Read the model definition and answer for the solid it produces. Units are mm, in the model's axes. A direction names the side the tool comes from. Round coordinates to 2 decimals unless told otherwise and drop trailing zeros. Order: outer loops, then holes, each group sorted by start corner. A loop starts at its lowest first (then second) coordinate and runs counter-clockwise, first axis right, second up. Notation, with made-up numbers: (2.5, 1) - (34.5, 1) arc R20 ccw to (34.5, 27) - close; hole circle Ø2 at (88, -31.75). An arc over 180 degrees is marked (long way). Answer as a JSON object with one key per item and string values. Group by question number.
Q1. A tool of negligible diameter and unlimited length cuts with its end or side. For faces 1 (the flat face through (-27, -12, 12)), 2 (the flat face through (-0.1, 10.2, 20)), 3 (the flat face through (27, -12, 12)), from which of +Z, -Z, +X, -X, +Y, -Y can it reach the whole face along a straight path? Write none if from no direction.
Q2. A cutting plane is placed at C-C on z = 1.5. Determine the outline of the cut face in (x, y).
Q3. A cutting plane is placed at D-D on y = -11. Determine the outline of the cut face in (x, z), and give its area (3 significant figures).
Q4. A cutting plane is placed at A-A on y = 0. Determine the outline of the cut face in (x, z), and give its area (3 significant figures).
Q5. A cutting plane is placed at B-B on x = 0. Determine the outline of the cut face in (y, z).
Q6. The mould has two halves that part along X. Classify faces 4 (the flat face through (30, -15, 12)), 5 (the flat face through (0, -8, 0)), 6 (the cylindrical face through (11.923, 3.755, 22.535)): pulls with the +X half, pulls with the -X half, needs draft (parallel to the pull), parting line crosses it, or undercut.
Q7. Given pin 1 Ø4 at (x, y) = (-21, -9.5) entering from +Z; pin 2 Ø1.5 at (x, z) = (10, 18.5) entering from +Y; pin 3 Ø7.5 at (x, y) = (-0.5, 3) entering from +Z; pin 4 Ø4 at (x, z) = (27.5, 9) entering from +Y, each flat-ended and moving along its own axis, determine where each tip first touches the part or whether it passes through.
Q8. Consider line 1 (Y direction, x = 0, z = 21.05); line 2 (Y direction, x = 0, z = 14.25); line 3 (Y direction, x = -26, z = 15.5). Determine where each line is inside the solid, lowest interval first.
```python
from build123d import *

# Parameters (mm, degrees)
F1_DEPTH       = 25
F2_R           = 10
F4_D           = 20
F4_DEPTH       = 22
F4_CBORE_D     = 25
F4_CBORE_DEPTH = 5
F4_TIP         = 6.0086061903


with BuildPart() as f1:
    # F0 (on Top) → F1 (new body)
    with BuildSketch(Plane.XY):
        with BuildLine():
            Line((9, -12), (-9, -12))
            ThreePointArc((-9, -12), (0, -15), (9, -12))
        make_face()
        with BuildLine():
            ThreePointArc((9, -12), (0, -15), (-9, -12))
            Line((-9, -12), (-30, -12))
            Line((-30, -12), (-30, -17))
            Line((-30, -17), (30, -17))
            Line((30, -17), (30, -12))
            Line((30, -12), (9, -12))
        make_face()
        with BuildLine():
            ThreePointArc((9, -12), (13.416407865, -6.7082039325), (15, 0))
            ThreePointArc((15, 0), (-6.7082039325, 13.416407865), (-9, -12))
            Line((-9, -12), (9, -12))
        make_face()
    extrude(amount=F1_DEPTH)

    # F2
    f2_edges = [f1.edges().sort_by_distance(p)[0] for p in [
        (-9, -12, 12.5),
        (9, -12, 12.5),
    ]]
    fillet(f2_edges, radius=F2_R)

    # F4
    with Locations(Plane.XY.offset(25)):
        with Locations((0, 0)):
            CounterBoreHole(F4_D / 2, F4_CBORE_D / 2, F4_CBORE_DEPTH, depth=F4_DEPTH)
            with Locations((0, 0, -(F4_DEPTH + F4_TIP / 2))):  # 118° drill point
                Cone(0, F4_D / 2, F4_TIP, mode=Mode.SUBTRACT)


solid = f1.part
```
Result set:
{
 "1": {"face 1": "+Z, -Z, -X, +Y", "face 2": "+Z", "face 3": "+Z, -Z, +X, +Y"},
 "2": {"outline": "(-30, -17) - (30, -17) - (30, -12) - (24.92, -12) arc R10 cw to (14.95, -1.2) arc R15 ccw (long way) to (-14.95, -1.2) arc R10 cw to (-24.92, -12) - (-30, -12) - close; hole circle Ø15.01 at (0, 0)"},
 "3": {"outline": "(-20.56, 0) - (20.56, 0) - (20.56, 25) - (5.94, 25) - (5.94, 20) - (-5.94, 20) - (-5.94, 25) - (-20.56, 25) - close", "area": "969 mm²"},
 "4": {"outline": "(-15, 0) - (-5.01, 0) - (-10, 3) - (-10, 20) - (-12.5, 20) - (-12.5, 25) - (-15, 25) - close; (5.01, 0) - (15, 0) - (15, 25) - (12.5, 25) - (12.5, 20) - (10, 20) - (10, 3) - close", "area": "240 mm²"},
 "5": {"outline": "(-17, 0) - (-5.01, 0) - (-10, 3) - (-10, 20) - (-12.5, 20) - (-12.5, 25) - (-17, 25) - close; (5.01, 0) - (15, 0) - (15, 25) - (12.5, 25) - (12.5, 20) - (10, 20) - (10, 3) - close"},
 "6": {"face 4": "pulls with the +X half", "face 5": "needs draft", "face 6": "undercut"},
 "7": {"pin 1": "stops at z = 25", "pin 2": "stops at y = 11.81", "pin 3": "stops at z = 1.07", "pin 4": "stops at y = -12"},
 "8": {"line 1": "y = -17 to -12.5, 12.5 to 15", "line 2": "y = -17 to -10, 10 to 15", "line 3": "y = -17 to -12"}
}
